from build123d import *

# Parameters (mm, degrees)
F1_DEPTH      = 4.5
F2_R          = 7
F3_DEPTH      = 10
F4_R          = 2.05
F5_DEPTH      = 25
F6_W          = 5
F6_H          = 1.9
F7_DEPTH      = 6
F8_R          = 1.6
F9_DEPTH      = 2.2693995383
F9_DEPTH_BACK = 25


with BuildPart() as f1:
    # F0 (on Top) → F1 (new body)
    with BuildSketch(Plane.XY):
        with BuildLine():
            ThreePointArc((3.3244697782, 13.0842615647), (2.806807826, 13.2049926099), (2.284794361, 13.3052513966))
            ThreePointArc((2.284794361, 13.3052513966), (0, 16.82), (-2.284794361, 13.3052513966))
            ThreePointArc((-2.284794361, 13.3052513966), (-2.806807826, 13.2049926099), (-3.3244697782, 13.0842615647))
            ThreePointArc((-3.3244697782, 13.0842615647), (-6.8413103365, 15.3658345975), (-7.4989967985, 11.2256423877))
            ThreePointArc((-7.4989967985, 11.2256423877), (-7.9351009059, 10.9217294241), (-8.3589028909, 10.6008840414))
            ThreePointArc((-8.3589028909, 10.6008840414), (-12.4996959645, 11.254776799), (-11.4165545633, 7.2050178281))
            ThreePointArc((-11.4165545633, 7.2050178281), (-11.6913429511, 6.75), (-11.9480057555, 6.2845173614))
            ThreePointArc((-11.9480057555, 6.2845173614), (-15.9967706041, 5.1976658454), (-13.3600863279, 1.9385802306))
            ThreePointArc((-13.3600863279, 1.9385802306), (-13.4260455875, 1.4111342541), (-13.4711898808, 0.8815005365))
            ThreePointArc((-13.4711898808, 0.8815005365), (-16.7278582801, -1.7581687522), (-12.9935377939, -3.6630555003))
            ThreePointArc((-12.9935377939, -3.6630555003), (-12.83926297, -4.1717294241), (-12.6650828937, -4.6739357393))
            ThreePointArc((-12.6650828937, -4.6739357393), (-14.5665472917, -8.41), (-10.3802885327, -8.6313156574))
            ThreePointArc((-10.3802885327, -8.6313156574), (-10.0324551439, -9.0332631858), (-9.6690680157, -9.4212060644))
            ThreePointArc((-9.6690680157, -9.4212060644), (-9.8865479436, -13.6076658454), (-5.9721930823, -12.1071429242))
            ThreePointArc((-5.9721930823, -12.1071429242), (-5.4909446815, -12.3328636782), (-5.001183437, -12.539464272))
            ThreePointArc((-5.001183437, -12.539464272), (-3.4970746396, -16.4524426443), (-0.5314511923, -13.4895351896))
            ThreePointArc((-0.5314511923, -13.4895351896), (0, -13.5), (0.5314511923, -13.4895351896))
            ThreePointArc((0.5314511923, -13.4895351896), (3.4970746396, -16.4524426443), (5.001183437, -12.539464272))
            ThreePointArc((5.001183437, -12.539464272), (5.4909446815, -12.3328636782), (5.9721930823, -12.1071429242))
            ThreePointArc((5.9721930823, -12.1071429242), (9.8865479436, -13.6076658454), (9.6690680157, -9.4212060644))
            ThreePointArc((9.6690680157, -9.4212060644), (10.0324551439, -9.0332631858), (10.3802885327, -8.6313156574))
            ThreePointArc((10.3802885327, -8.6313156574), (14.5665472917, -8.41), (12.6650828937, -4.6739357393))
            ThreePointArc((12.6650828937, -4.6739357393), (12.83926297, -4.1717294241), (12.9935377939, -3.6630555003))
            ThreePointArc((12.9935377939, -3.6630555003), (16.7278582801, -1.7581687522), (13.4711898808, 0.8815005365))
            ThreePointArc((13.4711898808, 0.8815005365), (13.4260455875, 1.4111342541), (13.3600863279, 1.9385802306))
            ThreePointArc((13.3600863279, 1.9385802306), (15.9967706041, 5.1976658454), (11.9480057555, 6.2845173614))
            ThreePointArc((11.9480057555, 6.2845173614), (11.6913429511, 6.75), (11.4165545633, 7.2050178281))
            ThreePointArc((11.4165545633, 7.2050178281), (12.4996959645, 11.254776799), (8.3589028909, 10.6008840414))
            ThreePointArc((8.3589028909, 10.6008840414), (7.9351009059, 10.9217294241), (7.4989967985, 11.2256423877))
            ThreePointArc((7.4989967985, 11.2256423877), (6.8413103365, 15.3658345975), (3.3244697782, 13.0842615647))
        make_face()
    extrude(amount=F1_DEPTH)

    # F2 (on face) → F3 (join)
    with BuildSketch(Plane.XY.offset(4.5)):
        Circle(F2_R)
    extrude(amount=F3_DEPTH)

    # F4 (on face) → F5 (cut)
    with BuildSketch(Plane.XY.offset(14.5)):
        Circle(F4_R)
    extrude(amount=-F5_DEPTH, mode=Mode.SUBTRACT)

    # F6 (on face) → F7 (cut)
    with BuildSketch(Plane.XY.offset(14.5)):
        with Locations((0, 4.5)):
            Rectangle(F6_W, F6_H)
    extrude(amount=-F7_DEPTH, mode=Mode.SUBTRACT)

    # F8 (on face) → F9 (cut, two sides)
    with BuildSketch(Plane(origin=(0, 3.55, 0), x_dir=(-1, 0, 0), z_dir=(0, 1, 0))) as f9_sk:
        with Locations((0, 11.5)):
            Circle(F8_R)
    extrude(amount=-F9_DEPTH, mode=Mode.SUBTRACT)
    extrude(f9_sk.sketch, amount=F9_DEPTH_BACK, mode=Mode.SUBTRACT)


solid = f1.part
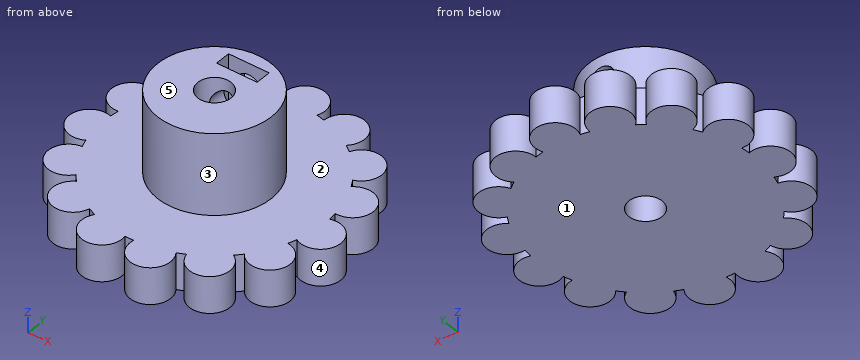
CAD build for the part. Positions are in the model's coordinates, mm. Face numbers are marked on the shaded views. A direction names the side the tool comes from. Coordinates: 2 decimals unless noted, no trailing zeros. Write each loop counter-clockwise with the first axis right and the second up, starting at its lowest first coordinate (ties: lowest second). Pieces come first, ordered by that corner, then holes. Notation, with made-up numbers: M 19,-17.5 L 70,-17.5 A22 ccw 70,-1.5 Z; hole C 38.5,-35 d11. An arc over 180 degrees is marked long. Answer as a JSON object with one key per item and string values. Group by question number.
1) Saw through at D-D (y = 0). Write the cut outline in (x, z), plus the area to 3 significant figures.
2) Tool access for the marked faces 1 and 2: list every direction of +Z, -Z, +X, -X, +Y, -Y with a clear straight run to the whole face (end or side of a thin tool).
3) Saw through at C-C (y = 14.32). Write the cut outline in (x, z), plus the area to 3 significant figures.
4) Mould opens along X. For the marked faces 3, 4 and 5 say: +X half, -X half, draft (parallel to the pull), parting line (faces both ways), or undercut.
5) Saw through at B-B (z = 9). Write the cut outline in (x, y), plus the area to 3 significant figures.
6) Saw through at A-A (x = 0). Write the cut outline in (y, z).
7) Pin check, flat tips, straight feed: pin 1 Ø2 at (x, y) = (10, 11.5) entering from +Z; pin 2 Ø6 at (x, z) = (0.5, 12) entering from +Y; pin 3 Ø5 at (x, z) = (0, 11.5) entering from -Y; pin 4 Ø16.5 at (x, y) = (-0.5, 8.5) entering from +Z. Stop position of each tip, or through.
8) Wall check: line 1 (X direction, y = -13, z = 1.75); line 2 (Z direction, x = 0, y = 6); line 3 (Y direction, x = 0, z = 5.5). Give the ranges that are in metal, low to high. Write a range as from..to.
Values follow:
{
 "1": {"outline": "M -16.24,0 L -2.05,0 L -2.05,14.5 L -7,14.5 L -7,4.5 L -16.24,4.5 Z; M 2.05,0 L 16.24,0 L 16.24,4.5 L 7,4.5 L 7,14.5 L 2.05,14.5 Z", "area": "227 mm2"},
 "2": {"face 1": "-Z, +X, -X, +Y, -Y", "face 2": "+Z"},
 "3": {"outline": "M -8,0 L -3.65,0 L -3.65,4.5 L -8,4.5 Z; M -2.5,0 L 2.5,0 L 2.5,4.5 L -2.5,4.5 Z; M 3.65,0 L 8,0 L 8,4.5 L 3.65,4.5 Z", "area": "61.6 mm2"},
 "4": {"face 3": "parting line", "face 4": "undercut", "face 5": "draft"},
 "5": {"outline": "C 0,0 d14; hole M -2.5,3.55 L 2.5,3.55 L 2.5,5.45 L -2.5,5.45 Z; hole C 0,0 d4.1", "area": "131 mm2"},
 "6": {"outline": "M -13.5,0 L -2.05,0 L -2.05,14.5 L -7,14.5 L -7,4.5 L -13.5,4.5 Z; M 2.05,0 L 16.82,0 L 16.82,4.5 L 7,4.5 L 7,9.9 L 5.45,9.9 L 5.45,8.5 L 3.55,8.5 L 3.55,9.9 L 2.05,9.9 Z; M 2.05,13.1 L 3.55,13.1 L 3.55,14.5 L 2.05,14.5 Z; M 5.45,13.1 L 7,13.1 L 7,14.5 L 5.45,14.5 Z"},
 "7": {"pin 1": "stops at z = 4.5", "pin 2": "stops at y = 7", "pin 3": "stops at y = -7", "pin 4": "stops at z = 14.5"},
 "8": {"line 1": "x = -10.48..-6.36, -5.27..5.27, 6.36..10.48", "line 2": "z = 0..9.9, 13.1..14.5", "line 3": "y = -7..-2.05, 2.05..7"}
}
